Work out the finished part from the listing and answer in its coordinate system (mm). Round coordinates to 2 decimals unless told otherwise and drop trailing zeros. Order: outer loops, then holes, each group sorted by start corner. A loop starts at its lowest first (then second) coordinate and runs counter-clockwise, first axis right, second up. Notation, with made-up numbers: M -4.5,67 L 12.5,67 A10 cw 12.5,74 Z; hole C -19,10 d8. An arc over 180 degrees is marked long. Return JSON: item names as keys, results as strings.
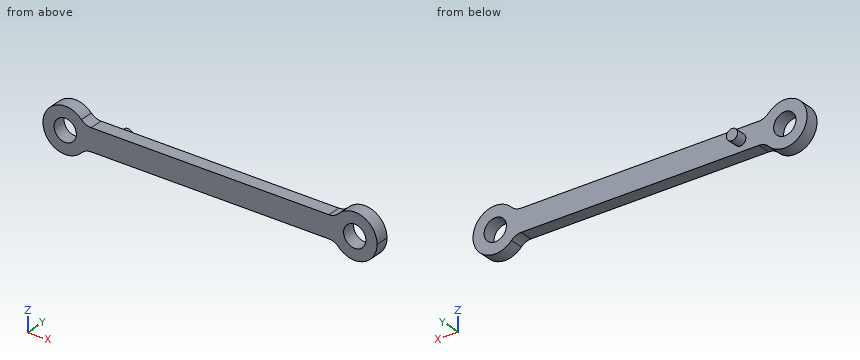
from build123d import *

# Parameters (mm, degrees)
EXTRUDE_1_DEPTH     = 6
FILLET_1_R          = 6
SKETCH_2_R          = 5
CUT_EXTRUDE_1_DEPTH = 6
SKETCH_3_R          = 2.5
EXTRUDE_2_DEPTH     = 5


with BuildPart() as part:
    # 草图1 → 凸台-拉伸1 (new body)
    with BuildSketch(Plane(origin=(0, 0, 0), x_dir=(1, 0, 0), z_dir=(0, 1, 0))):
        with BuildLine():
            Line((0, 5), (0, 0))
            Line((0, 0), (0, -5))
            Line((0, -5), (8.660254038, -5))
            ThreePointArc((8.660254038, -5), (9.659258263, -2.588190451), (10, 0))
            ThreePointArc((10, 0), (9.659258263, 2.588190451), (8.660254038, 5))
            Line((8.660254038, 5), (0, 5))
        make_face()
        with BuildLine():
            Line((0, -5), (0, 0))
            Line((0, 0), (0, 5))
            Line((0, 5), (8.660254038, 5))
            ThreePointArc((8.660254038, 5), (-10, 0), (8.660254038, -5))
            Line((8.660254038, -5), (0, -5))
        make_face()
        with BuildLine():
            ThreePointArc((10, 0), (9.659258263, -2.588190451), (8.660254038, -5))
            Line((8.660254038, -5), (121.339745962, -5))
            ThreePointArc((121.339745962, -5), (120, 0), (121.339745962, 5))
            Line((121.339745962, 5), (8.660254038, 5))
            ThreePointArc((8.660254038, 5), (9.659258263, 2.588190451), (10, 0))
        make_face()
        with BuildLine():
            Line((0, 5), (0, 0))
            Line((0, 0), (0, -5))
            Line((0, -5), (8.660254038, -5))
            ThreePointArc((8.660254038, -5), (9.659258263, -2.588190451), (10, 0))
            ThreePointArc((10, 0), (9.659258263, 2.588190451), (8.660254038, 5))
            Line((8.660254038, 5), (0, 5))
        make_face()
        with BuildLine():
            Line((0, -5), (0, 0))
            Line((0, 0), (0, 5))
            Line((0, 5), (8.660254038, 5))
            ThreePointArc((8.660254038, 5), (-10, 0), (8.660254038, -5))
            Line((8.660254038, -5), (0, -5))
        make_face()
        with BuildLine():
            ThreePointArc((121.339745962, 5), (120, 0), (121.339745962, -5))
            Line((121.339745962, -5), (130, -5))
            Line((130, -5), (130, 5))
            Line((130, 5), (121.339745962, 5))
        make_face()
        with BuildLine():
            Line((130, -5), (121.339745962, -5))
            ThreePointArc((121.339745962, -5), (132.588190451, -9.659258263), (140, 0))
            ThreePointArc((140, 0), (132.588190451, 9.659258263), (121.339745962, 5))
            Line((121.339745962, 5), (130, 5))
            Line((130, 5), (130, -5))
        make_face()
        with BuildLine():
            ThreePointArc((121.339745962, 5), (120, 0), (121.339745962, -5))
            Line((121.339745962, -5), (130, -5))
            Line((130, -5), (130, 5))
            Line((130, 5), (121.339745962, 5))
        make_face()
        with BuildLine():
            Line((130, -5), (121.339745962, -5))
            ThreePointArc((121.339745962, -5), (132.588190451, -9.659258263), (140, 0))
            ThreePointArc((140, 0), (132.588190451, 9.659258263), (121.339745962, 5))
            Line((121.339745962, 5), (130, 5))
            Line((130, 5), (130, -5))
        make_face()
    extrude(amount=EXTRUDE_1_DEPTH)

    # 圆角1
    fillet_1_edges = [part.edges().sort_by_distance(p)[0] for p in [
        (8.660254038, 3, -5),
        (121.339745962, 3, -5),
        (121.339745962, 3, 5),
        (8.660254038, 3, 5),
    ]]
    fillet(fillet_1_edges, radius=FILLET_1_R)

    # 草图2 → 切除-拉伸1 (cut)
    with BuildSketch(Plane(origin=(0, 6, 0), x_dir=(1, 0, 0), z_dir=(0, 1, 0))):
        with Locations(Location((0, 0, 0), (0, 0, 270))):
            Circle(SKETCH_2_R)
        with Locations(Location((130, 0, 0), (0, 0, 270))):
            Circle(SKETCH_2_R)
    extrude(amount=-CUT_EXTRUDE_1_DEPTH, mode=Mode.SUBTRACT)

    # 草图3 → 凸台-拉伸2 (add)
    with BuildSketch(Plane(origin=(0, 6, 0), x_dir=(1, 0, 0), z_dir=(0, 1, 0))):
        with Locations(Location((20, 0, 0), (0, 0, 270))):
            Circle(SKETCH_3_R)
    extrude(amount=EXTRUDE_2_DEPTH)


solid = part.part
Item 1: Each of these flat-tipped pins is pushed along its axis until it touches: pin 1 (5 mm diameter, centred on y = 7, z = -4, fed in from -X); pin 2 (2 mm diameter, centred on y = 1.5, z = -8, fed in from -X); pin 3 (6 mm diameter, centred on x = 62, z = -4, fed in from +Y). Where does it stop, or does it pass through?
Output:
{"pin 1": "stops at x = -9.85", "pin 2": "stops at x = -7.14", "pin 3": "stops at y = 6"}
Item 2: Find section B-B (y = 4.5). Determine the outline of the cut face in (x, z) (3 decimals).
Output:
{"outline": "M 7.262,-6.875 A6 cw 11.619,-5 L 118.381,-5 A6 cw 122.738,-6.875 A10 ccw long 122.738,6.875 A6 cw 118.381,5 L 11.619,5 A6 cw 7.262,6.875 A10 ccw long Z; hole C 0,0 d10; hole C 130,0 d10"}
Item 3: Find section A-A (x = 0). Determine the outline of the cut face in (y, z).
Output:
{"outline": "M 0,-10 L 6,-10 L 6,-5 L 0,-5 Z; M 0,5 L 6,5 L 6,10 L 0,10 Z"}
Item 4: Find section D-D (x = 37.5). Determine the outline of the cut face in (y, z), plus the area to 3 significant figures.
Output:
{"outline": "M 0,-5 L 6,-5 L 6,5 L 0,5 Z", "area": "60.0 mm^2"}
Item 5: Find section C-C (x = 20). Determine the outline of the cut face in (y, z).
Output:
{"outline": "M 0,-5 L 6,-5 L 6,-2.5 L 11,-2.5 L 11,2.5 L 6,2.5 L 6,5 L 0,5 Z"}
Item 6: Consider line 1 along X through (y, z) = (1.5, -7); line 2 along X through (y, z) = (2.5, -8.75); line 3 along Y through (x, z) = (24, 0.25). Determine where each line is inside the solid, lowest interval first. Write a range as [from, to].
Output:
{"line 1": "x = [-7.14, 7.14], [122.86, 137.14]", "line 2": "x = [-4.84, 4.84], [125.16, 134.84]", "line 3": "y = [0, 6]"}
